from build123d import *

# Parameters (mm, degrees)
F0_W     = 16.51
F0_H     = 16.51
F0_W_2   = 13.208
F0_H_2   = 13.208
F1_DEPTH = 1.651
F0_W_3   = 10
F0_H_3   = 10
F2_DEPTH = 0.5588
F3_DEPTH = 1.397
F4_DEPTH = 1.524


with BuildPart() as f1:
    # F0 (on Top) → F1 (new body)
    with BuildSketch(Plane.XY):
        Rectangle(F0_W, F0_H)
        Rectangle(F0_W_2, F0_H_2, mode=Mode.SUBTRACT)
    extrude(amount=F1_DEPTH)

    # F0 (on Top) → F2 (join)
    with BuildSketch(Plane.XY):
        Rectangle(F0_W, F0_H)
        Rectangle(F0_W_2, F0_H_2, mode=Mode.SUBTRACT)
        Rectangle(F0_W_2, F0_H_2)
        Rectangle(F0_W_3, F0_H_3, mode=Mode.SUBTRACT)
        Rectangle(F0_W_3, F0_H_3)
    extrude(amount=F2_DEPTH)

    # F3 (add): a face of the model
    f3_faces = [f1.faces().sort_by_distance(p)[0] for p in [
        (0, 0, 0.5588),
    ]]
    extrude(f3_faces, amount=F3_DEPTH)

    # F0 (on Top) → F4 (join)
    with BuildSketch(Plane.XY):
        Rectangle(F0_W_3, F0_H_3)
    extrude(amount=F4_DEPTH)


solid = f1.part
Read the model definition and answer for the solid it produces. Units are mm, in the model's axes. Give positions to 0.01 mm unless a question says otherwise; leave off trailing zeros. Write each loop counter-clockwise with the first axis right and the second up, starting at its lowest first coordinate (ties: lowest second). Pieces come first, ordered by that corner, then holes. Notation, with made-up numbers: (72.25, -25.75) - (124.25, -25.75) arc R23 ccw to (124.25, -11.75) - close; hole circle Ø8 at (70.5, 44). An arc over 180 degrees is marked (long way). Use CSV: the item, a comma, the result in double quotes. Start each with the question number.
(1) Consider line 1 along Y through (x, z) = (-6.25, 1.8); line 2 along Z through (x, y) = (-7, 3.25). Determine where each line is inside the solid, lowest interval first.
(2) Find section A-A (x = 4.25). Give the vertices of the cut face in (y, z) (3 decimals).
Findings below:
1,line 1,"-6.6 to 6.6"
1,line 2,"0 to 1.65"
2,outline,"(-8.255, 0) - (8.255, 0) - (8.255, 1.651) - (6.604, 1.651) - (6.604, 1.956) - (-6.604, 1.956) - (-6.604, 1.651) - (-8.255, 1.651) - close"
